Design review of the part built by this model. Coordinates are the model's own, in mm. Face numbers are marked on the shaded views. Round coordinates to 2 decimals unless told otherwise and drop trailing zeros. Loops run counter-clockwise (first coordinate to the right, second up) from the corner with the lowest first, then second, coordinate; pieces in that order, holes last. Notation, with made-up numbers: (-18.75, 1) -> (-14.75, 1) arc R12 ccw to (-14.75, 24) -> close; hole circle Ø9 at (17, 8.25). An arc over 180 degrees is marked (long way). Use a Markdown table: item, result. Add a question column.
Autodesk Inventor part; units mm, degrees
ref_plane "YZ Plane" through (0, 0, 0) normal (1, 0, 0) x (0, 1, 0)
ref_plane "XZ Plane" through (0, 0, 0) normal (0, 1, 0) x (-1, 0, 0)
ref_plane "XY Plane" through (0, 0, 0) normal (0, 0, 1) x (1, 0, 0)
sketch "Sketch1" plane through (0, 0, 0) normal (0, 1, 0) x (-1, 0, 0)
  circle A0 centre (0, 0) radius 6.35
  dimension "d0" = 12.7
extrude "Extrusion1" add sketch "Sketch1" along normal blind 25.4
sketch "Sketch2" plane through (0, 25.4, 0) normal (0, 1, 0) x (1, 0, 0)
  point P0 (0, 0)
  point P1 (0, 0)
hole "Hole1" at (0, 25.4, 0) direction (0, -1, 0) diameter 6.35 end through all
chamfer "Chamfer1" distance 0.635 angle 45 2 edges at (6.35, 25.4, 0) (6.35, 0, 0)
chamfer "Chamfer2" distance 0.635 angle 45 2 edges at (0, 25.4, -3.175) (0, 0, -3.175)
properties part number "Practice_001_1inchspacer" material "Aluminum 6061"
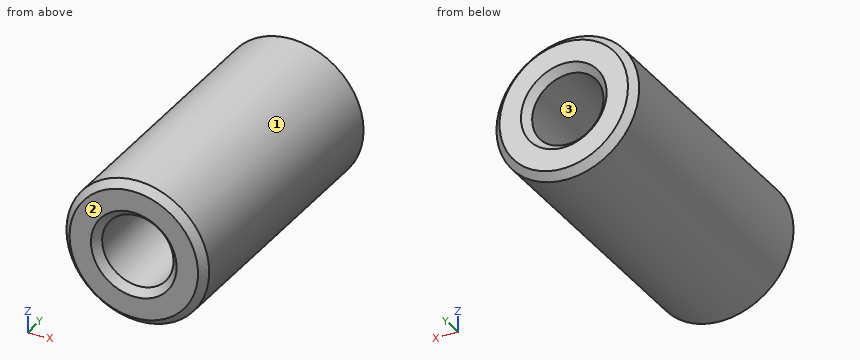
1. Mouldability with a two-part tool opening along X and no side actions: class the marked faces 1, 2 and 3 as +X half, -X half, draft (parallel to the pull), parting line (faces both ways), or undercut.
2. To check wall thickness, follow probe 1 along Z at (x, y) = (0, 6.75) (3 decimals); probe 2 along X at (y, z) = (19.5, 1.25); probe 3 along Z at (x, y) = (-2.75, 16.5). State the ranges of each line that lie inside material, in increasing order. Write a range as from..to.
3. Consider section C-C on y = 12.5. State the section outline as (x, z) points (3 decimals), plus the area to 3 significant figures.
4. Insertion check: P1, Ø1.5, axis at y = 10.5, z = 4.5, coming from the -X side; P2, Ø2, axis at x = 2, y = 13, coming from the -Z side; P3, Ø2, axis at y = 8, z = 2, coming from the -X side. Each pin has a flat end and moves straight along its axis. Give the tip position at first contact, or say it passes through.
5. Consider section A-A on x = 0. State the section outline as (y, z) points (3 decimals).
6. Consider section B-B on z = 0. State the section outline as (x, y) points (3 decimals), plus the area to 3 significant figures.
Verdict:
| question | item | result |
|---|---|---|
| 1 | face 1 | parting line |
| 1 | face 2 | draft |
| 1 | face 3 | undercut |
| 2 | probe 1 | z = -6.35..-3.175, 3.175..6.35 |
| 2 | probe 2 | x = -6.23..-2.92, 2.92..6.23 |
| 2 | probe 3 | z = -5.72..-1.59, 1.59..5.72 |
| 3 | outline | circle Ø12.7 at (0, 0); hole circle Ø6.35 at (0, 0) |
| 3 | area | 95.0 mm² |
| 4 | P1 | stops at x = -5.12 |
| 4 | P2 | stops at z = -6.27 |
| 4 | P3 | stops at x = -6.27 |
| 5 | outline | (0, -5.715) -> (0.635, -6.35) -> (24.765, -6.35) -> (25.4, -5.715) -> (25.4, -3.81) -> (24.765, -3.175) -> (0.635, -3.175) -> (0, -3.81) -> close; (0, 3.81) -> (0.635, 3.175) -> (24.765, 3.175) -> (25.4, 3.81) -> (25.4, 5.715) -> (24.765, 6.35) -> (0.635, 6.35) -> (0, 5.715) -> close |
| 6 | outline | (-6.35, 0.635) -> (-5.715, 0) -> (-3.81, 0) -> (-3.175, 0.635) -> (-3.175, 24.765) -> (-3.81, 25.4) -> (-5.715, 25.4) -> (-6.35, 24.765) -> close; (3.175, 0.635) -> (3.81, 0) -> (5.715, 0) -> (6.35, 0.635) -> (6.35, 24.765) -> (5.715, 25.4) -> (3.81, 25.4) -> (3.175, 24.765) -> close |
| 6 | area | 160 mm² |
